```python
from build123d import *

# Parameters (mm, degrees)
SKETCH1_W           = 25.4
SKETCH1_H           = 25.4
BOSS_EXTRUDE1_DEPTH = 25.4
FILLET1_R           = 5
SKETCH2_W           = 24.5
SKETCH2_H           = 24.5
BOSS_EXTRUDE2_DEPTH = 20
SKETCH3_W           = 22
SKETCH3_H           = 22
CUT_EXTRUDE1_DEPTH  = 20
SKETCH4_W           = 24.5
SKETCH4_H           = 24.5
BOSS_EXTRUDE3_DEPTH = 20
SKETCH5_W           = 22
SKETCH5_H           = 18
CUT_EXTRUDE2_DEPTH  = 23


with BuildPart() as part:
    # Sketch1 → Boss-Extrude1 (new body)
    with BuildSketch(Plane(origin=(0, 0, 0), x_dir=(1, 0, 0), z_dir=(0, 1, 0))):
        Rectangle(SKETCH1_W, SKETCH1_H)
    extrude(amount=BOSS_EXTRUDE1_DEPTH)

    # Fillet1
    fillet1_edges = [part.edges().sort_by_distance(p)[0] for p in [
        (-12.7, 25.4, 0),
    ]]
    fillet(fillet1_edges, radius=FILLET1_R)

    # Sketch2 → Boss-Extrude2 (add)
    with BuildSketch(Plane(origin=(12.7, 0, 0), x_dir=(0, 0, -1), z_dir=(1, 0, 0))):
        with Locations((0, 12.7)):
            Rectangle(SKETCH2_W, SKETCH2_H)
    extrude(amount=BOSS_EXTRUDE2_DEPTH)

    # Sketch3 → Cut-Extrude1 (cut)
    with BuildSketch(Plane(origin=(32.7, 0, 0), x_dir=(0, 0, -1), z_dir=(1, 0, 0))):
        with Locations((0, 12.7)):
            Rectangle(SKETCH3_W, SKETCH3_H)
    extrude(amount=-CUT_EXTRUDE1_DEPTH, mode=Mode.SUBTRACT)

    # Sketch4 → Boss-Extrude3 (add)
    with BuildSketch(Plane.XZ):
        Rectangle(SKETCH4_W, SKETCH4_H)
    extrude(amount=BOSS_EXTRUDE3_DEPTH)

    # Sketch5 → Cut-Extrude2 (cut)
    with BuildSketch(Plane(origin=(12.25, 0, 0), x_dir=(0, 0, -1), z_dir=(1, 0, 0))):
        with Locations((0, -10)):
            Rectangle(SKETCH5_W, SKETCH5_H)
    extrude(amount=-CUT_EXTRUDE2_DEPTH, mode=Mode.SUBTRACT)


solid = part.part
```
Verification items for the finished model (mm, model axes). A direction names the side the tool comes from. Round coordinates to 2 decimals unless told otherwise and drop trailing zeros. Write each loop counter-clockwise with the first axis right and the second up, starting at its lowest first coordinate (ties: lowest second). Pieces come first, ordered by that corner, then holes. Notation, with made-up numbers: (19, 50.25) -> (40, 50.25) arc R25 ccw to (40, 82.25) -> close; hole circle Ø8 at (69.5, 27). An arc over 180 degrees is marked (long way). Write each question's results on one line, items separated by ' | '. Start each with the question number.
1. Cross-section at D-D (x = 9). Enter the section's corners in (y, z).
2. Depth check by flat-ended pin: P1, Ø6, axis at x = -2, y = -10.5, coming from the +Z side; P2, Ø20, axis at x = 2, y = -12, coming from the -Z side; P3, Ø6, axis at x = 24, z = 1.5, coming from the -Y side; P4, Ø22, axis at x = 19, y = 10.5, coming from the +Z side. Enter the tip coordinate at first touch or a pass-through.
3. Material ranges on probe 1 along Y at (x, z) = (3.5, 10.75); probe 2 along Z at (x, y) = (-3.5, -14); probe 3 along Y at (x, z) = (17, 4), recorded low to high. Write a range as from..to.
4. Cross-section at A-A (x = 14). Enter the section's corners in (y, z), then the cut area to 3 significant figures.
5. Draft check along Y on faces 5 (the flat face through (23, 24.95, 0)), 6 (the flat face through (-12.25, -10, 0)), 7 (the flat face through (1, -10, -11)). Enter one of: +Y half, -Y half, draft (parallel to the pull), parting line (faces both ways), or undercut.
6. Cross-section at B-B (z = 5.5). Enter the section's corners in (x, y).
7. Set-up check for faces 1 (the flat face through (23, 13, -12.25)), 2 (the flat face through (23, 13, 12.25)), 3 (the flat face through (0, -10, -12.25)), 4 (the flat face through (23, 13, -11)): record each of +Z, -Z, +X, -X, +Y, -Y from which the full face is reachable in a straight line by a thin tool's end or side.
8. Cross-section at C-C (y = -4.5). Enter the section's corners in (x, z).
Solutions:
1) outline: (-20, -12.25) -> (0, -12.25) -> (0, -12.7) -> (25.4, -12.7) -> (25.4, 12.7) -> (0, 12.7) -> (0, 12.25) -> (-20, 12.25) -> close; hole (-19, -11) -> (-1, -11) -> (-1, 11) -> (-19, 11) -> close
2) P1: stops at z = 12.25 | P2: stops at z = -12.25 | P3: stops at y = 0.45 | P4: stops at z = 12.7
3) probe 1: y = -20..-19, -1..25.4 | probe 2: z = -12.25..-11, 11..12.25 | probe 3: y = 0.45..1.7, 23.7..24.95
4) outline: (0.45, -12.25) -> (24.95, -12.25) -> (24.95, 12.25) -> (0.45, 12.25) -> close; hole (1.7, -11) -> (23.7, -11) -> (23.7, 11) -> (1.7, 11) -> close | area: 116 mm2
5) face 5: +Y half | face 6: draft | face 7: undercut
6) outline: (-12.7, 0) -> (-12.25, 0) -> (-12.25, -20) -> (12.25, -20) -> (12.25, -19) -> (-10.75, -19) -> (-10.75, -1) -> (12.25, -1) -> (12.25, 0) -> (12.7, 0) -> (12.7, 0.45) -> (32.7, 0.45) -> (32.7, 1.7) -> (12.7, 1.7) -> (12.7, 23.7) -> (32.7, 23.7) -> (32.7, 24.95) -> (12.7, 24.95) -> (12.7, 25.4) -> (-7.7, 25.4) arc R5 ccw to (-12.7, 20.4) -> close
7) face 1: -Z, +X, +Y, -Y | face 2: +Z, +X, +Y, -Y | face 3: -Z, +X, -X, -Y | face 4: +X
8) outline: (-12.25, -12.25) -> (12.25, -12.25) -> (12.25, -11) -> (-10.75, -11) -> (-10.75, 11) -> (12.25, 11) -> (12.25, 12.25) -> (-12.25, 12.25) -> close
